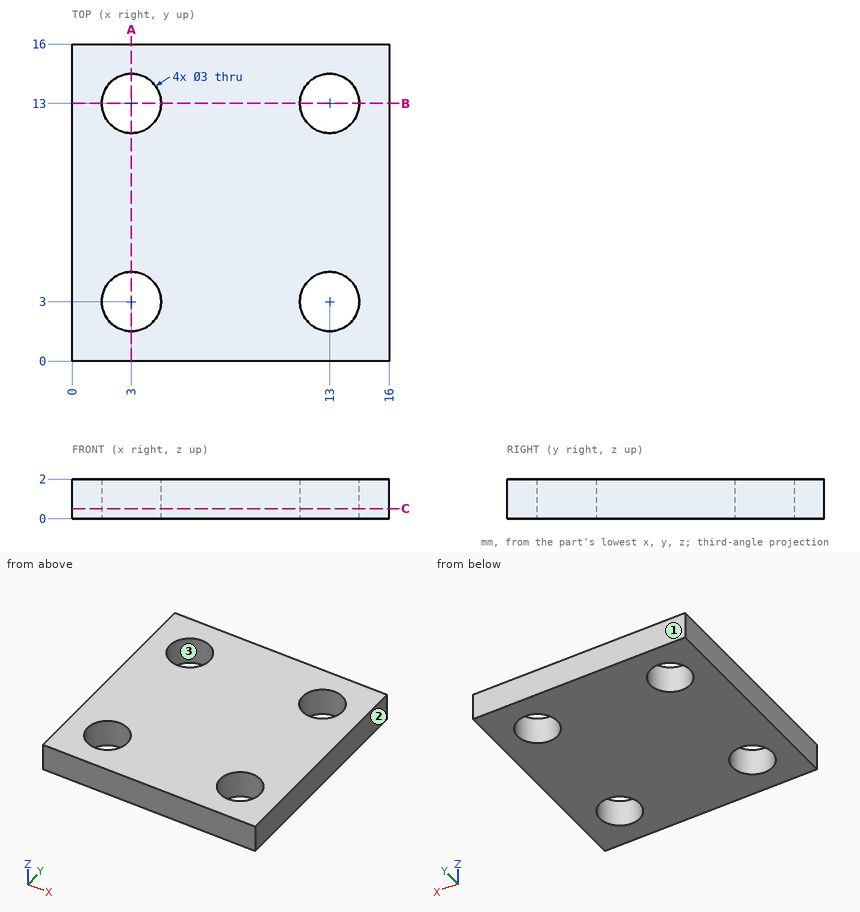
Source: three-view drawing plus pictorial views. Frame: mm from the lowest corner of the part. Round coordinates to 2 decimals unless told otherwise and drop trailing zeros. Loops run counter-clockwise (first coordinate to the right, second up) from the corner with the lowest first, then second, coordinate; pieces in that order, holes last. Notation, with made-up numbers: M -10.5,60.25 L 46.5,60.25 A14 cw 46.5,85.25 Z; hole C 87.5,-2.5 d5. An arc over 180 degrees is marked long. Answer as CSV lines item,"result". Start each with the question number.
(1) Section A-A, the plane x = 3. Output: boundary loops of the cut face in (y, z), plus the area to 3 significant figures.
(2) Draft query along Y for the marked faces 1, 2 and 3. Return one class per face: released by +Y, released by -Y, zero draft, split by the parting line, or undercut.
(3) Line query: line 1 (Y direction, x = 3, z = 1.5); line 2 (X direction, y = 11.75, z = 1.25). Output: solid intervals per line, ascending. Write a range as [from, to].
(4) Section C-C, the plane z = 0.5. Output: boundary loops of the cut face in (x, y), plus the area to 3 significant figures.
Values found:
1,outline,"M 0,0 L 1.5,0 L 1.5,2 L 0,2 Z; M 4.5,0 L 11.5,0 L 11.5,2 L 4.5,2 Z; M 14.5,0 L 16,0 L 16,2 L 14.5,2 Z"
1,area,"20.0 mm²"
2,face 1,"released by +Y"
2,face 2,"zero draft"
2,face 3,"undercut"
3,line 1,"y = [0, 1.5], [4.5, 11.5], [14.5, 16]"
3,line 2,"x = [0, 2.17], [3.83, 12.17], [13.83, 16]"
4,outline,"M 0,0 L 16,0 L 16,16 L 0,16 Z; hole C 3,3 d3; hole C 3,13 d3; hole C 13,3 d3; hole C 13,13 d3"
4,area,"228 mm²"
